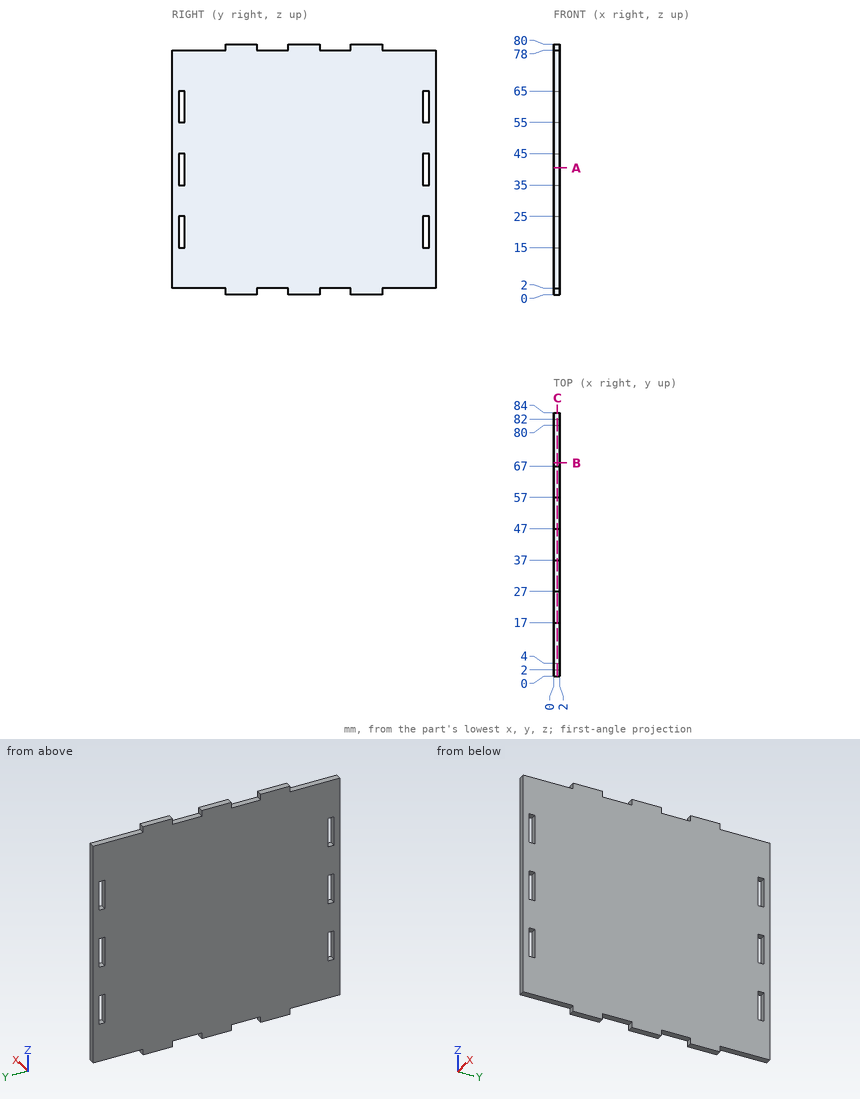
For this review, use the dimensioned drawing (mm, ordinates from the lowest corner) and the shaded views. Round coordinates to 2 decimals unless told otherwise and drop trailing zeros. Order: outer loops, then holes, each group sorted by start corner. A loop starts at its lowest first (then second) coordinate and runs counter-clockwise, first axis right, second up. Notation, with made-up numbers: M 9,61 L 21,61 A21 ccw 21,76 Z; hole C 17,-24.5 d4. An arc over 180 degrees is marked long. Write each question's results on one line, items separated by ' | '. Start each with the question number.
1. To check wall thickness, follow L1, parallel to Y at x = 1.4, z = 36; L2, parallel to Z at x = 0.9, y = 9.5. State the ranges of each line that lie inside material, in increasing order. Write a range as [from, to].
2. Add section B-B (y = 68). State the section outline as (x, z) points, then the cut area to 3 significant figures.
3. Add section A-A (z = 40.5). State the section outline as (x, y) points.
4. Add section C-C (x = 1.25). State how many separate pieces and enclosed holes the cut face has, then the cut area to 3 significant figures.
5. Clearance check with flat-ended pins moving along their axes: pin 1 Ø0.6 at (x, z) = (1, 78.5) entering from +Y; pin 2 Ø0.6 at (x, z) = (0.5, 78.5) entering from -Y; pin 3 Ø1 at (x, y) = (0.5, 3) entering from +Z. State where each tip first meets the part, or that it passes through.
Output values:
1) L1: [0, 2], [4, 80], [82, 84] | L2: [2, 78]
2) outline: M 0,2 L 2,2 L 2,78 L 0,78 Z | area: 152 mm^2
3) outline: M 0,0 L 2,0 L 2,2 L 0,2 Z; M 0,4 L 2,4 L 2,80 L 0,80 Z; M 0,82 L 2,82 L 2,84 L 0,84 Z
4) separate pieces: 1 | enclosed holes: 6 | area: 6,380 mm^2
5) pin 1: y = 67 | pin 2: y = 17 | pin 3: z = 78
